Part model, mm, in its own coordinate system. A direction names the side the tool comes from. Coordinates: 2 decimals unless noted, no trailing zeros. Order: outer loops, then holes, each group sorted by start corner. A loop starts at its lowest first (then second) coordinate and runs counter-clockwise, first axis right, second up.
```python
from build123d import *
from OCP.BRepFilletAPI import BRepFilletAPI_MakeChamfer

# Parameters (mm, degrees)
SKETCH1_W                                 = 80
SKETCH1_H                                 = 90
BOSS_EXTRUDE1_DEPTH                       = 8
SKETCH6_R                                 = 3
BOSS_EXTRUDE7_DEPTH                       = 8
SKETCH7_W                                 = 80
SKETCH7_H                                 = 90
SKETCH7_W_2                               = 64
SKETCH7_H_2                               = 74
BOSS_EXTRUDE2_DEPTH                       = 7
SKETCH10_W                                = 5
SKETCH10_H                                = 64
BOSS_EXTRUDE3_DEPTH                       = 2
LPATTERN1_COUNT                           = 2
LPATTERN1_PITCH                           = 37
LPATTERN1_COL_COUNT                       = 2
LPATTERN1_COL_PITCH                       = 37
CBORE_START                               = -1
CBORE_FOR_M5_HEX_HEAD_BOLT3_OUTLINE_R     = 2.75
CBORE_FOR_M5_HEX_HEAD_BOLT3_DEPTH         = 9
CBORE_START_2                             = 7.99
CBORE_FOR_M5_HEX_HEAD_BOLT3_2_OUTLINE_R   = 6.12
CBORE_FOR_M5_HEX_HEAD_BOLT3_2_OUTLINE_R_2 = 2.75
CBORE_FOR_M5_HEX_HEAD_BOLT3_2_DEPTH       = 0.01
SKETCH11_W                                = 5
SKETCH11_H                                = 74
BOSS_EXTRUDE4_DEPTH                       = 2
LPATTERN2_COUNT                           = 2
LPATTERN2_PITCH                           = 32
LPATTERN2_COL_COUNT                       = 2
LPATTERN2_COL_PITCH                       = 32
BOSS_EXTRUDE6_REACH                       = 123.347
SKETCH20_R                                = 8
CBORE_FOR_M5_HEX_HEAD_BOLT2_D             = 5.5
CBORE_FOR_M5_HEX_HEAD_BOLT2_CBORE_D       = 12.24
CBORE_FOR_M5_HEX_HEAD_BOLT2_CBORE_DEPTH   = 7
FILLET1_SIZE                              = 10
F_1_16_0_0625_DIAMETER_HOLE1_D            = 1.5875
F_1_16_0_0625_DIAMETER_HOLE1_DEPTH        = 11
F_1_16_0_0625_DIAMETER_HOLE1_TIP          = 0.476933116
CHAMFER1_SIZE                             = 2.5
CHAMFER1_SIZE2                            = 6.868693549


with BuildPart() as part:
    # Sketch1 → Boss-Extrude1 (new body)
    with BuildSketch(Plane(origin=(0, 0, 0), x_dir=(0, 0, -1), z_dir=(1, 0, 0))):
        with Locations((40, 45)):
            Rectangle(SKETCH1_W, SKETCH1_H)
    extrude(amount=BOSS_EXTRUDE1_DEPTH)

    # Sketch6 → Boss-Extrude7 (add)
    with BuildSketch(Plane(origin=(8, 0, 0), x_dir=(0, 0, -1), z_dir=(1, 0, 0))):
        with Locations(Location((27.3, 53.89, 0), (0, 0, 180))):
            Circle(SKETCH6_R)
        with Locations(Location((27.3, 36.11, 0), (0, 0, 180))):
            Circle(SKETCH6_R)
        with Locations(Location((52.7, 36.11, 0), (0, 0, 180))):
            Circle(SKETCH6_R)
        with Locations(Location((52.7, 53.89, 0), (0, 0, 180))):
            Circle(SKETCH6_R)
    extrude(amount=BOSS_EXTRUDE7_DEPTH)

    # Sketch7 → Boss-Extrude2 (add)
    with BuildSketch(Plane(origin=(8, 0, 0), x_dir=(0, 0, -1), z_dir=(1, 0, 0))):
        with Locations((40, 45)):
            Rectangle(SKETCH7_W, SKETCH7_H)
        with Locations((40, 45)):
            Rectangle(SKETCH7_W_2, SKETCH7_H_2, mode=Mode.SUBTRACT)
    extrude(amount=BOSS_EXTRUDE2_DEPTH)

    # Sketch10 → Boss-Extrude3 (add, symmetric)
    with BuildSketch(Plane(origin=(0, 45, 0), x_dir=(1, 0, 0), z_dir=(0, 1, 0))):
        with Locations((10.5, 40)):
            Rectangle(SKETCH10_W, SKETCH10_H)
    boss_extrude3 = extrude(amount=BOSS_EXTRUDE3_DEPTH, both=True)

    # LPattern1: Boss-Extrude3 ×2
    with Locations(*[(0, i * LPATTERN1_PITCH, 0) for i in range(1, LPATTERN1_COUNT)]):
        add(boss_extrude3)

    # LPattern1 col: Boss-Extrude3 ×2
    with Locations(*[(0, -i * LPATTERN1_COL_PITCH, 0) for i in range(1, LPATTERN1_COL_COUNT)]):
        add(boss_extrude3)

    # CBORE for M5 Hex Head Bolt3: read off the stored shape, not the designer's step
    # CBORE for M5 Hex Head Bolt3 outline → CBORE for M5 Hex Head Bolt3 (cut)
    with BuildSketch(Plane.YZ.offset(CBORE_START)):
        with Locations((72, -52.5)):
            Circle(CBORE_FOR_M5_HEX_HEAD_BOLT3_OUTLINE_R)
        with Locations((18, -27.5)):
            Circle(CBORE_FOR_M5_HEX_HEAD_BOLT3_OUTLINE_R)
        with Locations((18, -52.5)):
            Circle(CBORE_FOR_M5_HEX_HEAD_BOLT3_OUTLINE_R)
        with Locations((72, -27.5)):
            Circle(CBORE_FOR_M5_HEX_HEAD_BOLT3_OUTLINE_R)
    extrude(amount=CBORE_FOR_M5_HEX_HEAD_BOLT3_DEPTH, mode=Mode.SUBTRACT)

    # CBORE for M5 Hex Head Bolt3 2 outline → CBORE for M5 Hex Head Bolt3 2 (cut)
    # profile 1 of 4: a face of its own
    with BuildSketch(Plane.YZ.offset(CBORE_START_2)):
        with Locations((72, -52.5)):
            Circle(CBORE_FOR_M5_HEX_HEAD_BOLT3_2_OUTLINE_R)
        with Locations((72, -52.5)):
            Circle(CBORE_FOR_M5_HEX_HEAD_BOLT3_2_OUTLINE_R_2, mode=Mode.SUBTRACT)
    # profile 2 of 4: a face of its own
    with BuildSketch(Plane.YZ.offset(CBORE_START_2)):
        with Locations((18, -27.5)):
            Circle(CBORE_FOR_M5_HEX_HEAD_BOLT3_2_OUTLINE_R)
        with Locations((18, -27.5)):
            Circle(CBORE_FOR_M5_HEX_HEAD_BOLT3_2_OUTLINE_R_2, mode=Mode.SUBTRACT)
    # profile 3 of 4: a face of its own
    with BuildSketch(Plane.YZ.offset(CBORE_START_2)):
        with Locations((18, -52.5)):
            Circle(CBORE_FOR_M5_HEX_HEAD_BOLT3_2_OUTLINE_R)
        with Locations((18, -52.5)):
            Circle(CBORE_FOR_M5_HEX_HEAD_BOLT3_2_OUTLINE_R_2, mode=Mode.SUBTRACT)
    # profile 4 of 4: a face of its own
    with BuildSketch(Plane.YZ.offset(CBORE_START_2)):
        with Locations((72, -27.5)):
            Circle(CBORE_FOR_M5_HEX_HEAD_BOLT3_2_OUTLINE_R)
        with Locations((72, -27.5)):
            Circle(CBORE_FOR_M5_HEX_HEAD_BOLT3_2_OUTLINE_R_2, mode=Mode.SUBTRACT)
    extrude(amount=CBORE_FOR_M5_HEX_HEAD_BOLT3_2_DEPTH, mode=Mode.SUBTRACT)

    # Sketch11 → Boss-Extrude4 (add, symmetric)
    with BuildSketch(Plane(origin=(0, 0, -40), x_dir=(-1, 0, 0), z_dir=(0, 0, -1))):
        with Locations((-10.5, 45)):
            Rectangle(SKETCH11_W, SKETCH11_H)
    boss_extrude4 = extrude(amount=BOSS_EXTRUDE4_DEPTH, both=True)

    # LPattern2: Boss-Extrude4 ×2
    with Locations(*[(0, 0, i * LPATTERN2_PITCH) for i in range(1, LPATTERN2_COUNT)]):
        add(boss_extrude4)

    # LPattern2 col: Boss-Extrude4 ×2
    with Locations(*[(0, 0, -i * LPATTERN2_COL_PITCH) for i in range(1, LPATTERN2_COL_COUNT)]):
        add(boss_extrude4)

    # Sketch20 → Boss-Extrude6 (add, up to next)
    with BuildSketch(Plane(origin=(15, 0, 0), x_dir=(0, 0, -1), z_dir=(1, 0, 0)), mode=Mode.PRIVATE) as boss_extrude6_sk1:
        with Locations((8, 82)):
            Circle(SKETCH20_R)
    boss_extrude6_tool1 = extrude(boss_extrude6_sk1.sketch, amount=-BOSS_EXTRUDE6_REACH, mode=Mode.PRIVATE) - part.part
    # Sketch20 → Boss-Extrude6 (add, up to next)
    with BuildSketch(Plane(origin=(15, 0, 0), x_dir=(0, 0, -1), z_dir=(1, 0, 0)), mode=Mode.PRIVATE) as boss_extrude6_sk2:
        with Locations((72, 82)):
            Circle(SKETCH20_R)
    boss_extrude6_tool2 = extrude(boss_extrude6_sk2.sketch, amount=-BOSS_EXTRUDE6_REACH, mode=Mode.PRIVATE) - part.part
    # Sketch20 → Boss-Extrude6 (add, up to next)
    with BuildSketch(Plane(origin=(15, 0, 0), x_dir=(0, 0, -1), z_dir=(1, 0, 0)), mode=Mode.PRIVATE) as boss_extrude6_sk3:
        with Locations((8, 8)):
            Circle(SKETCH20_R)
    boss_extrude6_tool3 = extrude(boss_extrude6_sk3.sketch, amount=-BOSS_EXTRUDE6_REACH, mode=Mode.PRIVATE) - part.part
    # Sketch20 → Boss-Extrude6 (add, up to next)
    with BuildSketch(Plane(origin=(15, 0, 0), x_dir=(0, 0, -1), z_dir=(1, 0, 0)), mode=Mode.PRIVATE) as boss_extrude6_sk4:
        with Locations((72, 8)):
            Circle(SKETCH20_R)
    boss_extrude6_tool4 = extrude(boss_extrude6_sk4.sketch, amount=-BOSS_EXTRUDE6_REACH, mode=Mode.PRIVATE) - part.part
    add(boss_extrude6_tool1.solids().sort_by_distance((15, 82, -8))[0])
    add(boss_extrude6_tool2.solids().sort_by_distance((15, 82, -72))[0])
    add(boss_extrude6_tool3.solids().sort_by_distance((15, 8, -8))[0])
    add(boss_extrude6_tool4.solids().sort_by_distance((15, 8, -72))[0])

    # CBORE for M5 Hex Head Bolt2 (through all)
    with Locations(Plane.ZY):
        with Locations((-8, 82), (-72, 82), (-8, 8), (-72, 8)):
            CounterBoreHole(CBORE_FOR_M5_HEX_HEAD_BOLT2_D / 2, CBORE_FOR_M5_HEX_HEAD_BOLT2_CBORE_D / 2, CBORE_FOR_M5_HEX_HEAD_BOLT2_CBORE_DEPTH)

    # Fillet1
    # a fillet whose section is not a circle: 10 mm, written as the material it takes off along each edge
    with BuildSketch(Plane(origin=(-25, 0, -80), x_dir=(0, 0, 1), z_dir=(1, 0, 0)), Plane(origin=(40, 0, 0), x_dir=(0, 0, -1), z_dir=(-1, 0, 0)), Plane(origin=(40, 90, 0), x_dir=(0, -1, 0), z_dir=(-1, 0, 0)), Plane(origin=(-25, 90, -80), x_dir=(0, -1, 0), z_dir=(1, 0, 0))) as fillet1_piece_1:
        with BuildLine():
            add(Edge.make_bspline([(FILLET1_SIZE, 0), (FILLET1_SIZE * 0.831801948466, 0), (FILLET1_SIZE * 0.663603896932, 0), (FILLET1_SIZE * 0.292893218813, -FILLET1_SIZE * 0.0716919198361), (FILLET1_SIZE * 0.0716919198361, -FILLET1_SIZE * 0.292893218813), (0, -FILLET1_SIZE * 0.663603896932), (0, -FILLET1_SIZE * 0.831801948466), (0, -FILLET1_SIZE)], knots=[0, 0, 0, 0, 0, 0, 0.5, 0.5, 1, 1, 1, 1, 1, 1], degree=5))
            Line((0, -FILLET1_SIZE), (0, 0))
            Line((0, 0), (FILLET1_SIZE, 0))
        make_face()
    extrude(amount=65, mode=Mode.SUBTRACT)

    # 1/16 (0.0625) Diameter Hole1
    with Locations(Plane(origin=(16, 0, 0), x_dir=(0, 0, -1), z_dir=(1, 0, 0))):
        with Locations((27.3, 53.89), (52.7, 53.89), (52.7, 36.11), (27.3, 36.11)):
            Hole(F_1_16_0_0625_DIAMETER_HOLE1_D / 2, depth=F_1_16_0_0625_DIAMETER_HOLE1_DEPTH)
            with Locations((0, 0, -(F_1_16_0_0625_DIAMETER_HOLE1_DEPTH + F_1_16_0_0625_DIAMETER_HOLE1_TIP / 2))):  # 118° drill point
                Cone(0, F_1_16_0_0625_DIAMETER_HOLE1_D / 2, F_1_16_0_0625_DIAMETER_HOLE1_TIP, mode=Mode.SUBTRACT)

    # Chamfer1: one chamfer whose edges measure the first distance from different faces: ONE call of the kernel's chamfer builder (chamfer() names one face for all edges)
    chamfer1_edges_1 = [part.edges().sort_by_distance(p)[0] for p in [
        (8, 53.89, -30.3),
    ]]
    chamfer1_side_1 = [part.faces().sort_by_distance(p)[0] for p in [
        (8, 62.109672107, -23.682631382),
    ]]
    chamfer1_edges_2 = [part.edges().sort_by_distance(p)[0] for p in [
        (8, 36.11, -30.3),
    ]]
    chamfer1_side_2 = [part.faces().sort_by_distance(p)[0] for p in [
        (8, 27.890327893, -23.682631382),
    ]]
    chamfer1_edges_3 = [part.edges().sort_by_distance(p)[0] for p in [
        (8, 36.11, -55.7),
    ]]
    chamfer1_side_3 = [part.faces().sort_by_distance(p)[0] for p in [
        (8, 27.890327893, -56.317368618),
    ]]
    chamfer1_edges_4 = [part.edges().sort_by_distance(p)[0] for p in [
        (8, 53.89, -55.7),
    ]]
    chamfer1_side_4 = [part.faces().sort_by_distance(p)[0] for p in [
        (8, 62.109672107, -56.317368618),
    ]]
    chamfer1 = BRepFilletAPI_MakeChamfer(part.part.solid().wrapped)
    for e in chamfer1_edges_1:
        chamfer1.Add(CHAMFER1_SIZE, CHAMFER1_SIZE2, e.wrapped, chamfer1_side_1[0].wrapped)  # the first distance lies on this face
    for e in chamfer1_edges_2:
        chamfer1.Add(CHAMFER1_SIZE, CHAMFER1_SIZE2, e.wrapped, chamfer1_side_2[0].wrapped)  # the first distance lies on this face
    for e in chamfer1_edges_3:
        chamfer1.Add(CHAMFER1_SIZE, CHAMFER1_SIZE2, e.wrapped, chamfer1_side_3[0].wrapped)  # the first distance lies on this face
    for e in chamfer1_edges_4:
        chamfer1.Add(CHAMFER1_SIZE, CHAMFER1_SIZE2, e.wrapped, chamfer1_side_4[0].wrapped)  # the first distance lies on this face
    add(Compound.cast(chamfer1.Shape()), mode=Mode.REPLACE)


solid = part.part
```
(1) Slice it at A-A, the plane y = 18. State how many separate pieces and enclosed holes the cut face has, then the cut area to 3 significant figures.
(2) Slice it at B-B, the plane z = -63. Give the cut face in (x, y).
(3) Drop flat-ended pins along their axis: pin 1 (7.5 mm diameter, centred on y = 82, z = -72, fed in from +X); pin 2 (1 mm diameter, centred on y = 68.5, z = -52.5, fed in from +X); pin 3 (10 mm diameter, centred on y = 31.5, z = -41.5, fed in from +X); pin 4 (4.5 mm diameter, centred on y = 18, z = -52.5, fed in from -X). Give the stop position or say it passes through.
(4) Probe line 1 (Y direction, x = 10.75, z = -19); line 2 (Z direction, x = 12, y = 48); line 3 (Y direction, x = 7.5, z = -52.7). List the from-to ranges inside material, lowest first.
(5) Tool access for faces 1 (the face through (8, 27, -24)), 2 (the face through (11.06, 6.95, -10.54)), 3 (the face through (7, 79, -71)): list every direction of +Z, -Z, +X, -X, +Y, -Y with a clear straight run to the whole face (end or side of a thin tool).
Here are the results:
1. separate pieces: 3
1. enclosed holes: 0
1. area: 704 mm2
2. outline: (0, 0) - (15, 0) - (15, 8) - (13, 8) - (13, 10) - (8, 10) - (8, 43) - (13, 43) - (13, 47) - (8, 47) - (8, 80) - (13, 80) - (13, 82) - (15, 82) - (15, 90) - (0, 90) - close
3. pin 1: stops at x = 15
3. pin 2: stops at x = 7.99
3. pin 3: stops at x = 13
3. pin 4: passes through
4. line 1: y = 0 to 10, 43 to 47, 80 to 90
4. line 2: z = -80 to -70, -42 to -38, -10 to 0
4. line 3: y = 0 to 15.26, 20.74 to 35.32, 36.9 to 53.1, 54.68 to 69.26, 74.74 to 90
5. face 1: +X
5. face 2: +X, -X
5. face 3: -X
